For this review, use the dimensioned drawing (mm, ordinates from the lowest corner) and the shaded views. Give positions to 0.01 mm unless a question says otherwise; leave off trailing zeros. Write each loop counter-clockwise with the first axis right and the second up, starting at its lowest first coordinate (ties: lowest second). Pieces come first, ordered by that corner, then holes. Notation, with made-up numbers: M -28.75,36 L -16.75,36 A24 ccw -16.75,55 Z; hole C -9,24 d8. An arc over 180 degrees is marked long. One line per item, written item: value. Start each with the question number.
Item 1: Consider section D-D, the plane z = 5. Write out the cut boundary in (x, y).
Item 2: To check wall thickness, follow probe 1 along Z at (x, y) = (1.9, 4.6); probe 2 along Y at (x, z) = (3.7, 10); probe 3 along Y at (x, z) = (3.35, 4). State the ranges of each line that lie inside material, in increasing order.
Item 3: Consider section A-A, the plane y = 2.5. Write out the cut boundary in (x, z), and give its area (3 significant figures).
Item 4: Consider section B-B, the plane z = 14. Write out the cut boundary in (x, y), and give its area (3 significant figures).
Item 5: Clearance check with a flat-ended pin moving along its axis: pin 1 Ø2 at (x, z) = (4.5, 3) entering from -Y. State where the tip first meets the part, or that it passes through.
Item 6: Consider section C-C, the plane x = 1.23. Write out the cut boundary in (y, z).
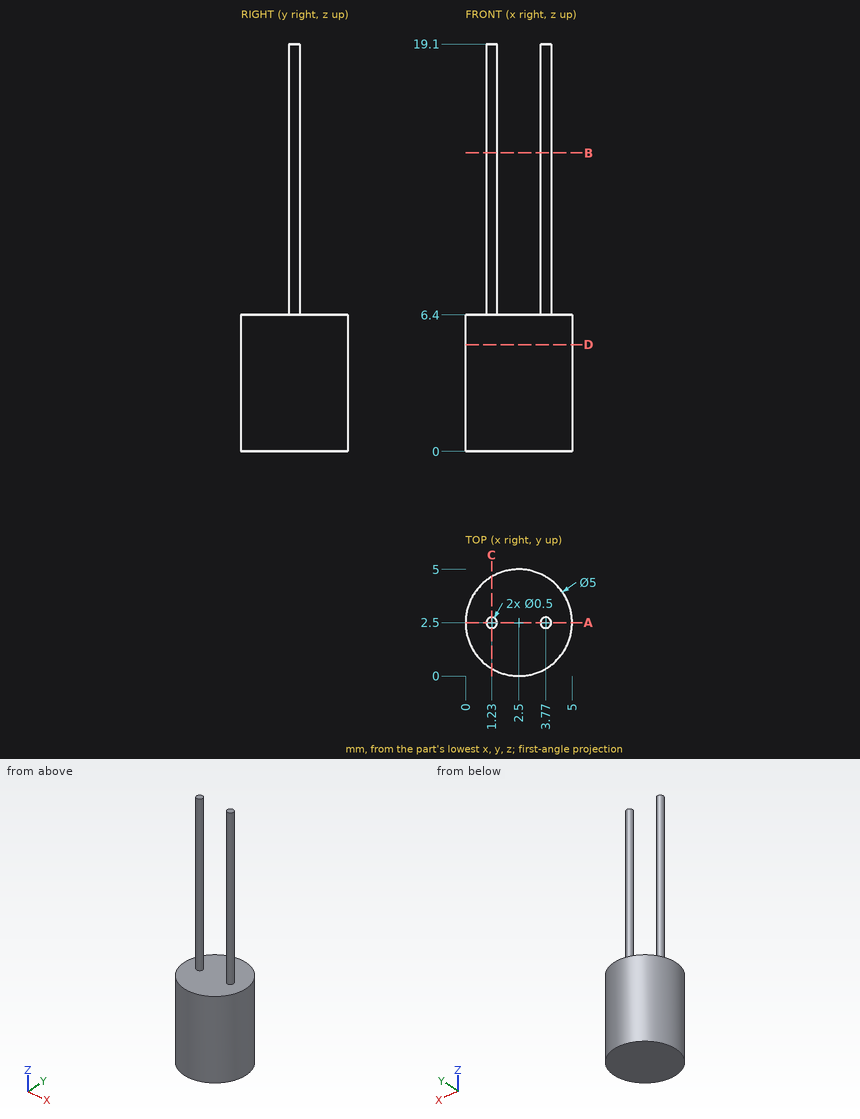
Model answer:
1. outline: C 2.5,2.5 d5
2. probe 1: z = 0 to 6.4
2. probe 2: y = 2.26 to 2.74
2. probe 3: y = 0.15 to 4.85
3. outline: M 0,0 L 5,0 L 5,6.4 L 4.02,6.4 L 4.02,19.1 L 3.52,19.1 L 3.52,6.4 L 1.48,6.4 L 1.48,19.1 L 0.98,19.1 L 0.98,6.4 L 0,6.4 Z
3. area: 44.7 mm2
4. outline: C 1.23,2.5 d0.5; C 3.77,2.5 d0.5
4. area: 0.393 mm2
5. pin 1: stops at y = 0.21
6. outline: M 0.35,0 L 4.65,0 L 4.65,6.4 L 2.75,6.4 L 2.75,19.1 L 2.25,19.1 L 2.25,6.4 L 0.35,6.4 Z
